from build123d import *

# Parameters (mm, degrees)
F0_W      = 39
F0_H      = 50
F0_R      = 3.5
F0_R_2    = 1.725
F1_DEPTH  = 4
F2_R      = 3.5
F3_DEPTH  = 2
F5_DEPTH  = 22
F6_R      = 5.25
F6_R_2    = 1.725
F7_DEPTH  = 6
F8_W      = 39
F8_H      = 50
F9_DEPTH  = 4
F10_R     = 1.99999
F11_R     = 1.725
F12_DEPTH = 4
F14_DEPTH = 2


# Not quite as in the source:
# - a fillet or chamfer is up to 0.001 mm smaller than in the source, because OpenCascade refuses the exact size


with BuildPart() as f1:
    # F0 (on Top) → F1 (new body)
    with BuildSketch(Plane.XY):
        with Locations((19.5, 25)):
            Rectangle(F0_W, F0_H)
        with Locations((9.5, 15)):
            Circle(F0_R, mode=Mode.SUBTRACT)
        with Locations((29.5, 15)):
            Circle(F0_R, mode=Mode.SUBTRACT)
        with Locations((9.5, 35)):
            Circle(F0_R, mode=Mode.SUBTRACT)
        with Locations((29.5, 35)):
            Circle(F0_R, mode=Mode.SUBTRACT)
        with Locations((9.5, 35)):
            Circle(F0_R)
        with Locations((9.5, 35)):
            Circle(F0_R_2, mode=Mode.SUBTRACT)
        with Locations((29.5, 35)):
            Circle(F0_R)
        with Locations((29.5, 35)):
            Circle(F0_R_2, mode=Mode.SUBTRACT)
        with Locations((29.5, 15)):
            Circle(F0_R)
        with Locations((29.5, 15)):
            Circle(F0_R_2, mode=Mode.SUBTRACT)
        with Locations((9.5, 15)):
            Circle(F0_R)
        with Locations((9.5, 15)):
            Circle(F0_R_2, mode=Mode.SUBTRACT)
    extrude(amount=F1_DEPTH)

    # F2 (on face) → F3 (cut)
    with BuildSketch(Plane.XY.offset(4)):
        with Locations((9.5, 35)):
            Circle(F2_R)
        with Locations((29.5, 35)):
            Circle(F2_R)
        with Locations((29.5, 15)):
            Circle(F2_R)
        with Locations((9.5, 15)):
            Circle(F2_R)
    extrude(amount=-F3_DEPTH, mode=Mode.SUBTRACT)

    # F4 (on face) → F5 (join)
    with BuildSketch(Plane.XY.offset(4)):
        Polygon((4, 50), (0, 50), (0, 0), (39, 0), (39, 50), (35, 50), (35, 6), (4, 6), align=None)
    extrude(amount=F5_DEPTH)

    # F6 (on face) → F7 (cut, through all)
    with BuildSketch(Plane(origin=(0, 6, 0), x_dir=(-1, 0, 0), z_dir=(0, 1, 0))):
        with Locations((-19.5, 15)):
            Circle(F6_R)
        with Locations((-27.1, 15)):
            Circle(F6_R_2)
        with Locations((-11.9, 15)):
            Circle(F6_R_2)
    extrude(amount=-F7_DEPTH, mode=Mode.SUBTRACT)

    # F8 (on face) → F9 (join)
    with BuildSketch(Plane.XY.offset(26)):
        with Locations((19.5, 25)):
            Rectangle(F8_W, F8_H)
    extrude(amount=F9_DEPTH)

    # F10 (radius 2 in the source; OpenCascade refuses exactly that, so slightly less here)
    f10_edges = [f1.edges().sort_by_distance(p)[0] for p in [
        (0, 25, 30),
        (0, 25, 0),
        (39, 25, 0),
        (39, 25, 30),
        (35, 28, 26),
        (4, 28, 26),
        (4, 28, 4),
        (35, 28, 4),
    ]]
    fillet(f10_edges, radius=F10_R)

    # F11 (on face) → F12 (cut, through all)
    with BuildSketch(Plane.XY.offset(30)):
        with Locations((9.5, 35)):
            Circle(F11_R)
        with Locations((29.5, 35)):
            Circle(F11_R)
        with Locations((29.5, 15)):
            Circle(F11_R)
        with Locations((9.5, 15)):
            Circle(F11_R)
    extrude(amount=-F12_DEPTH, mode=Mode.SUBTRACT)

    # F13 (on face) → F14 (cut)
    with BuildSketch(Plane(origin=(0, 0, 26), x_dir=(1, 0, 0), z_dir=(0, 0, -1))):
        Polygon((12.26, -13.406513257), (9.5, -11.8130265141), (6.74, -13.406513257), (6.74, -16.593486743), (9.5, -18.1869734859), (12.26, -16.593486743), align=None)
        Polygon((32.26, -13.406513257), (29.5, -11.8130265141), (26.74, -13.406513257), (26.74, -16.593486743), (29.5, -18.1869734859), (32.26, -16.593486743), align=None)
        Polygon((32.26, -33.406513257), (29.5, -31.8130265141), (26.74, -33.406513257), (26.74, -36.593486743), (29.5, -38.1869734859), (32.26, -36.593486743), align=None)
        Polygon((12.26, -33.406513257), (9.5, -31.8130265141), (6.74, -33.406513257), (6.74, -36.593486743), (9.5, -38.1869734859), (12.26, -36.593486743), align=None)
    extrude(amount=-F14_DEPTH, mode=Mode.SUBTRACT)


solid = f1.part
Build history of the part. All positions in model axes, mm. A direction names the side the tool comes from. Round coordinates to 2 decimals unless told otherwise and drop trailing zeros. Order: outer loops, then holes, each group sorted by start corner. A loop starts at its lowest first (then second) coordinate and runs counter-clockwise, first axis right, second up. Notation, with made-up numbers: M 26,-21 L 59,-21 A13 cw 59,-16 Z; hole C -39.75,29 d8. An arc over 180 degrees is marked long. Use CSV: the item, a comma, the result in double quotes. Start each with the question number.
(1) Cut at A-A on z = 11. List the corners of the cut face in (x, y).
(2) Mould opens along Z. For faces 4 (the face through (0.57, 25.35, 29.4)), 5 (the face through (32.26, 15, 27)), 6 (the face through (30.3, 33.47, 29.01)) say: +Z half, -Z half, draft (parallel to the pull), parting line (faces both ways), or undercut.
(3) Cut at D-D on z = 5.25. List the corners of the cut face in (x, y).
(4) Cut at B-B on y = 23.5. List the corners of the cut face in (x, z), then the cut area to 3 significant figures.
(5) Cut at C-C on y = 35. State how many separate pieces and enclosed holes the cut face has, then the cut area to 3 significant figures.
(6) Flat gauge pins, fed straight in: P1, Ø2, axis at x = 27.1, z = 15, coming from the +Y side; P2, Ø8, axis at x = 29, z = 13.5, coming from the +Y side. Where does each tip first touch, or does it go through?
(7) Tool access for faces 1 (the face through (31.145, 15.518, 0.986)), 2 (the face through (10.9, 12.62, 26.99)), 3 (the face through (4.57, 28.31, 25.4)): list every direction of +Z, -Z, +X, -X, +Y, -Y with a clear straight run to the whole face (end or side of a thin tool).
(8) Drill centre lines: probe 1 along Y at (x, z) = (9.5, 28.7) (3 decimals); probe 2 along Y at (x, z) = (29.5, 3.25); probe 3 along X at (y, z) = (32.5, 11.5). Where is each one in solid material? Low to high.
Findings:
1,outline,"M 0,0 L 16.1,0 L 16.1,6 L 4,6 L 4,50 L 0,50 Z; M 22.9,0 L 39,0 L 39,50 L 35,50 L 35,6 L 22.9,6 Z"
2,face 4,"+Z half"
2,face 5,"undercut"
2,face 6,"draft"
3,outline,"M 0,0 L 39,0 L 39,50 L 34.85,50 L 34.85,6 L 4.15,6 L 4.15,50 L 0,50 Z"
4,outline,"M 0,2 A2 ccw 2,0 L 37,0 A2 ccw 39,2 L 39,28 A2 ccw 37,30 L 2,30 A2 ccw 0,28 Z; hole M 4,6 A2 ccw 6,4 L 33,4 A2 ccw 35,6 L 35,24 A2 ccw 33,26 L 6,26 A2 ccw 4,24 Z"
4,area,"488 mm^2"
5,separate pieces,"4"
5,enclosed holes,"0"
5,area,"410 mm^2"
6,P1,"passes through"
6,P2,"stops at y = 6"
7,face 1,"+Z, -Z"
7,face 2,"none"
7,face 3,"+Y"
8,probe 1,"y = 0 to 13.275, 16.725 to 33.275, 36.725 to 50"
8,probe 2,"y = 0 to 11.5, 18.5 to 31.5, 38.5 to 50"
8,probe 3,"x = 0 to 4, 35 to 39"
